from build123d import *

# Parameters (mm, degrees)
SKETCH_1_R          = 1.6
SKETCH_1_R_2        = 2
SKETCH_1_R_3        = 1.5
SKETCH_1_R_4        = 1.4
SKETCH_1_R_5        = 2.65
EXTRUDE_1_DEPTH     = 3
EXTRUDE_START       = -3
SKETCH_2_R          = 2
EXTRUDE_2_DEPTH     = 3
SKETCH_3_R          = 2
CUT_EXTRUDE_1_DEPTH = 292.701502722


with BuildPart() as part:
    # 草图1 → 凸台-拉伸1 (new body)
    with BuildSketch(Plane.XY):
        with BuildLine():
            Line((180.876359785, 205.228138488), (168.831228405, 205.268129507))
            ThreePointArc((168.831228405, 205.268129507), (167.414263571, 204.689029851), (166.821803423, 203.277599114))
            add(Edge.make_bspline(
                [(161.786060078, 195.71078825), (165.139642387, 198.941974737), (166.821803423, 203.277599114)],
                knots=[0, 0, 0, 1, 1, 1], degree=2))
            add(Edge.make_bspline(
                [(161.786060078, 195.71078825), (164.92793776, 192.361073548), (166.750316725, 188.143977385)],
                knots=[0, 0, 0, 1, 1, 1], degree=2))
            ThreePointArc((166.750316725, 188.143977385), (167.329416381, 186.727012552), (168.740847117, 186.134552403))
            Line((168.740847117, 186.134552403), (178.027494719, 186.090685063))
            ThreePointArc((178.027494719, 186.090685063), (181.763769971, 184.38667788), (182.963862725, 180.459443405))
            Line((182.963862725, 180.459443405), (173.564244058, 106.60839258))
            ThreePointArc((173.564244058, 106.60839258), (173.458389771, 106.114066832), (173.271035356, 105.644533662))
            Line((173.271035356, 105.644533662), (156.40182897, 71.937427408))
            ThreePointArc((156.40182897, 71.937427408), (156.165380125, 71.54355997), (155.871567565, 71.190411567))
            Line((155.871567565, 71.190411567), (142.35670304, 57.268944585))
            ThreePointArc((142.35670304, 57.268944585), (141.191974376, 55.555727126), (140.679319548, 53.548517136))
            ThreePointArc((140.679319548, 53.548517136), (140.625900814, 52.473146463), (140.63043091, 51.396459358))
            ThreePointArc((140.63043091, 51.396459358), (141.098279223, 49.25350905), (142.305067834, 47.421903384))
            Line((142.305067834, 47.421903384), (155.331422881, 33.891052634))
            ThreePointArc((155.331422881, 33.891052634), (157.115873944, 32.615571364), (159.239509549, 32.066672572))
            ThreePointArc((159.239509549, 32.066672572), (160.240879339, 32.022528199), (161.243203239, 32.028609273))
            ThreePointArc((161.243203239, 32.028609273), (163.386153547, 32.496457586), (165.217759213, 33.703246197))
            Line((165.217759213, 33.703246197), (178.748609963, 46.729601244))
            ThreePointArc((178.748609963, 46.729601244), (180.024091234, 48.514052307), (180.572990025, 50.637687912))
            ThreePointArc((180.572990025, 50.637687912), (180.619914226, 52.200895683), (180.544552467, 53.762990758))
            ThreePointArc((180.544552467, 53.762990758), (180.310185029, 54.977736199), (179.831664348, 56.118592254))
            Line((179.831664348, 56.118592254), (174.566586824, 65.746386199))
            ThreePointArc((174.566586824, 65.746386199), (174.20435551, 67.001908028), (174.410236103, 68.292318726))
            Line((174.410236103, 68.292318726), (186.173266888, 97.935631449))
            ThreePointArc((186.173266888, 97.935631449), (186.3010118, 98.338133742), (186.37097439, 98.754585534))
            Line((186.37097439, 98.754585534), (194.807070925, 186.357605284))
            ThreePointArc((194.807070925, 186.357605284), (195.598752445, 188.613890348), (197.347624572, 190.244543041))
            Line((197.347624572, 190.244543041), (199.704104393, 191.559498626))
            ThreePointArc((199.704104393, 191.559498626), (199.85169861, 191.684777969), (199.940640273, 191.856732461))
            Line((199.940640273, 191.856732461), (204.447932197, 207.383938176))
            ThreePointArc((204.447932197, 207.383938176), (204.348738584, 207.847132715), (203.907590711, 208.019693161))
            Line((203.907590711, 208.019693161), (180.876359785, 205.228138488))
        make_face()
        with Locations((160.943625523, 69.015853918)):
            Circle(SKETCH_1_R, mode=Mode.SUBTRACT)
        with Locations((177.617675606, 51.696037122)):
            Circle(SKETCH_1_R, mode=Mode.SUBTRACT)
        with Locations((160.29785881, 35.02198704)):
            Circle(SKETCH_1_R, mode=Mode.SUBTRACT)
        with Locations((176.600254281, 99.006041366)):
            Circle(SKETCH_1_R_2, mode=Mode.SUBTRACT)
        with Locations((174.2076694, 89.744683982)):
            Circle(SKETCH_1_R_2, mode=Mode.SUBTRACT)
        with Locations((188.100780779, 175.340948835)):
            Circle(SKETCH_1_R_3, mode=Mode.SUBTRACT)
        with Locations((193.30497456, 194.25027454)):
            Circle(SKETCH_1_R_2, mode=Mode.SUBTRACT)
        with Locations((177.198714362, 196.226687268)):
            Circle(SKETCH_1_R_2, mode=Mode.SUBTRACT)
        with Locations((143.623808727, 52.341803836)):
            Circle(SKETCH_1_R, mode=Mode.SUBTRACT)
        with Locations((166.515909108, 45.895440526)):
            Circle(SKETCH_1_R_4, mode=Mode.SUBTRACT)
        with Locations((166.744222119, 57.91408742)):
            Circle(SKETCH_1_R_4, mode=Mode.SUBTRACT)
        with Locations((154.497262214, 46.123753537)):
            Circle(SKETCH_1_R_4, mode=Mode.SUBTRACT)
        with Locations((154.725575225, 58.142400432)):
            Circle(SKETCH_1_R_4, mode=Mode.SUBTRACT)
        with Locations((160.620742166, 52.018920479)):
            Circle(SKETCH_1_R_5, mode=Mode.SUBTRACT)
        with BuildLine():
            Line((188.440185855, 163.909601849), (185.367574986, 166.984339314))
            ThreePointArc((185.367574986, 166.984339314), (184.827033477, 167.094676686), (184.513989502, 166.640404821))
            Line((184.513989502, 166.640404821), (184.414122911, 161.383318097))
            ThreePointArc((184.414122911, 161.383318097), (184.67712622, 160.933508785), (185.197409188, 160.961877628))
            Line((185.197409188, 160.961877628), (188.369886648, 163.144226888))
            ThreePointArc((188.369886648, 163.144226888), (188.584414353, 163.510438603), (188.440185855, 163.909601849))
        make_face(mode=Mode.SUBTRACT)
        with BuildLine():
            Line((187.472818663, 156.632762387), (183.440770681, 153.85911402))
            ThreePointArc((183.440770681, 153.85911402), (183.226691028, 153.497542793), (183.363942447, 153.100395594))
            Line((183.363942447, 153.100395594), (187.266298258, 149.046906048))
            ThreePointArc((187.266298258, 149.046906048), (187.809036476, 148.928189955), (188.126412768, 149.384184004))
            Line((188.126412768, 149.384184004), (188.25610494, 156.211321918))
            ThreePointArc((188.25610494, 156.211321918), (187.99310163, 156.66113123), (187.472818663, 156.632762387))
        make_face(mode=Mode.SUBTRACT)
        with BuildLine():
            Line((182.20568655, 146.790661355), (182.089798545, 140.690189901))
            ThreePointArc((182.089798545, 140.690189901), (182.344789249, 140.244786653), (182.857830944, 140.2586622))
            Line((182.857830944, 140.2586622), (186.260617668, 142.420502707))
            ThreePointArc((186.260617668, 142.420502707), (186.486525093, 142.765499158), (186.376380029, 143.162896669))
            Line((186.376380029, 143.162896669), (183.08948131, 147.101527616))
            ThreePointArc((183.08948131, 147.101527616), (182.539690059, 147.252837448), (182.20568655, 146.790661355))
        make_face(mode=Mode.SUBTRACT)
        with BuildLine():
            Line((185.171612374, 137.402888306), (181.107941286, 132.130958638))
            ThreePointArc((181.107941286, 132.130958638), (181.008086118, 131.761532658), (181.198701468, 131.429700776))
            Line((181.198701468, 131.429700776), (185.105024507, 128.418656815))
            ThreePointArc((185.105024507, 128.418656815), (185.626655398, 128.363912237), (185.910183153, 128.805169268))
            Line((185.910183153, 128.805169268), (186.067531203, 137.088142897))
            ThreePointArc((186.067531203, 137.088142897), (185.733347108, 137.569375609), (185.171612374, 137.402888306))
        make_face(mode=Mode.SUBTRACT)
        with BuildLine():
            Line((183.984397253, 122.483643411), (180.383752933, 126.798230005))
            ThreePointArc((180.383752933, 126.798230005), (179.833961683, 126.949539837), (179.499958174, 126.487363744))
            Line((179.499958174, 126.487363744), (179.363127608, 119.284452918))
            ThreePointArc((179.363127608, 119.284452918), (179.638411409, 118.828253811), (180.168779422, 118.879327956))
            Line((180.168779422, 118.879327956), (183.906254307, 121.767652188))
            ThreePointArc((183.906254307, 121.767652188), (184.097560783, 122.109032943), (183.984397253, 122.483643411))
        make_face(mode=Mode.SUBTRACT)
        with BuildLine():
            Line((183.611833626, 116.147486542), (178.84837762, 112.466283102))
            ThreePointArc((178.84837762, 112.466283102), (178.655459645, 112.107236418), (178.793914924, 111.723880183))
            Line((178.793914924, 111.723880183), (182.801955086, 107.560613253))
            ThreePointArc((182.801955086, 107.560613253), (183.326638992, 107.435215573), (183.659857408, 107.85945992))
            Line((183.659857408, 107.85945992), (184.415273253, 115.703930291))
            ThreePointArc((184.415273253, 115.703930291), (184.159230917, 116.189582633), (183.611833626, 116.147486542))
        make_face(mode=Mode.SUBTRACT)
    extrude(amount=EXTRUDE_1_DEPTH)

    # 草图2 → 凸台-拉伸2 (add)
    with BuildSketch(Plane.XY.offset(3).offset(EXTRUDE_START)):
        with Locations((193.30497456, 194.25027454)):
            Circle(SKETCH_2_R)
    extrude(amount=EXTRUDE_2_DEPTH)

    # 草图3 → 切除-拉伸1 (cut, through all)
    with BuildSketch(Plane.XY.offset(3)):
        with Locations((190.164017385, 195.374410179)):
            Circle(SKETCH_3_R)
    extrude(amount=-CUT_EXTRUDE_1_DEPTH, mode=Mode.SUBTRACT)


solid = part.part
Check sheet for the modelled part. Datum: model origin and axes. Units: mm. A direction names the side the tool comes from. Give positions to 0.01 mm unless a question says otherwise; leave off trailing zeros. Order: outer loops, then holes, each group sorted by start corner. A loop starts at its lowest first (then second) coordinate and runs counter-clockwise, first axis right, second up. Notation, with made-up numbers: M 8,16 L 27,16 A24 cw 27,26 Z; hole C 86.25,49 d8. An arc over 180 degrees is marked long. Answer as CSV lines item,"result". Start each with the question number.
Item 1: Cross-section at B-B on x = 151.5. Enter the section's corners in (y, z).
Item 2: Cross-section at C-C on z = 1.75. State how many separate pieces and enclosed holes the cut face has, plus the area to 3 significant figures.
Item 3: Gauge pin test, flat ends, axial feed: P1, Ø1.8, axis at x = 188.1, y = 175.34, coming from the -Z side; P2, Ø5, axis at x = 176.6, y = 99.01, coming from the -Z side. Record the tip position at first contact, or that the pin passes through.
Item 4: Mould release check, pull along X, two halves, no side actions. Record for faces 1 (the face through (192.553, 206.643, 1.479)), 2 (the face through (183.12, 129.95, 1.48)), 3 (the face through (180.011, 48.486, 1.479)): +X half, -X half, draft (parallel to the pull), parting line (faces both ways), or undercut.
Item 5: Cross-section at A-A on y = 75. Enter the section's corners in (x, z).
Item 6: Tool access check on faces 4 (the face through (186.925, 165.425, 1.479)), 5 (the face through (177.236, 60.865, 1.479)), 6 (the face through (164.955, 89.027, 1.479)). Record the directions out of +Z, -Z, +X, -X, +Y, -Y that give a thin tool (end or side, any length) a straight path to the whole face; none if there is none.
Item 7: Thickness scan on line 1 (X direction, y = 59, z = 2.1); line 2 (X direction, y = 166, z = 1.3); line 3 (Y direction, x = 164.5, z = 2.4). Record the ranges inside material, lowest first. Write a range as [from, to].
Established:
1,outline,"M 37.87,0 L 66.69,0 L 66.69,3 L 37.87,3 Z"
2,separate pieces,"1"
2,enclosed holes,"20"
2,area,"3,130 mm^2"
3,P1,"passes through"
3,P2,"stops at z = 0"
4,face 1,"-X half"
4,face 2,"undercut"
4,face 3,"+X half"
5,outline,"M 157.93,0 L 177.07,0 L 177.07,3 L 157.93,3 Z"
6,face 4,"+Z, -Z"
6,face 5,"+Z, -Z, +X"
6,face 6,"+Z, -Z, -X"
7,line 1,"x = [144.04, 153.62], [155.83, 165.86], [167.63, 178.26]"
7,line 2,"x = [181.12, 184.5], [186.35, 192.85]"
7,line 3,"y = [33.11, 88.12], [192.29, 198.89]"
